Input: part model. Units: mm. Frame: model coordinates. Round coordinates to 2 decimals unless told otherwise and drop trailing zeros. Loops run counter-clockwise (first coordinate to the right, second up) from the corner with the lowest first, then second, coordinate; pieces in that order, holes last.
(1) First-contact query: pin 1 Ø8 at (x, y) = (35, -4) entering from +Z; pin 2 Ø6 at (y, z) = (9, -38) entering from -X; pin 3 Ø8 at (x, y) = (43, -3.5) entering from -Z. Flat tips, straight axial feed; report the tip coordinate or a pass-through.
(2) Cut plane A-A, the plane z = -40. Output: boundary loops of the cut face in (x, y), and give its area (3 significant figures).
(3) Cut plane B-B, the plane z = -23.5. Output: boundary loops of the cut face in (x, y), and give its area (3 significant figures).
(4) Line query: line 1 (X direction, y = 5.75, z = 1); line 2 (X direction, y = 3, z = 22); line 3 (Z direction, x = 27.5, y = 3.25). Output: solid intervals per line, ascending.
from build123d import *

# Parameters (mm, degrees)
F1_DEPTH = 12.7


with BuildPart() as f1:
    # F0 (on Front) → F1 (new body, symmetric)
    with BuildSketch(Plane.XZ):
        with BuildLine():
            ThreePointArc((-57.9073168337, 0), (0, -57.9073168337), (57.9073168337, 0))
            add(Edge.make_bspline(
                [(57.9073168337, 0), (57.7035928826, 5.0836857421), (57.2764841542, 15.9200002784), (62.591224193, 35.1555711006), (59.6648907409, 58.6163574282), (41.6811280162, 72.8568929301), (21.7803366448, 82.0664074952), (7.4388819921, 90.9145052404), (0, 95.504)],
                knots=[0, 0, 0, 0, 0.1433978074, 0.3056661676, 0.4767459335, 0.6452017867, 0.8159666021, 1, 1, 1, 1], degree=3))
            add(Edge.make_bspline(
                [(-57.9073168337, 0), (-57.7035928826, 5.0836857421), (-57.2764841542, 15.9200002784), (-62.591224193, 35.1555711006), (-59.6648907409, 58.6163574282), (-41.6811280162, 72.8568929301), (-21.7803366448, 82.0664074952), (-7.4388819921, 90.9145052404), (0, 95.504)],
                knots=[0, 0, 0, 0, 0.1433978074, 0.3056661676, 0.4767459335, 0.6452017867, 0.8159666021, 1, 1, 1, 1], degree=3))
        make_face()
    extrude(amount=F1_DEPTH, both=True)


solid = f1.part
Reported:
1. pin 1: stops at z = 77.79
1. pin 2: stops at x = -46.13
1. pin 3: stops at z = -42.8
2. outline: (-41.87, -12.7) - (41.87, -12.7) - (41.87, 12.7) - (-41.87, 12.7) - close
2. area: 2,130 mm2
3. outline: (-52.92, -12.7) - (52.92, -12.7) - (52.92, 12.7) - (-52.92, 12.7) - close
3. area: 2,690 mm2
4. line 1: x = -57.87 to 57.87
4. line 2: x = -59.17 to 59.17
4. line 3: z = -50.96 to 79.6
